For this review, take the finished solid that the model builds, in its own axes (mm). Face numbers are marked on the shaded views. A direction names the side the tool comes from. Coordinates: 2 decimals unless noted, no trailing zeros. Loops run counter-clockwise (first coordinate to the right, second up) from the corner with the lowest first, then second, coordinate; pieces in that order, holes last. Notation, with made-up numbers: M 1,-40 L 36,-40 A14 ccw 36,-31 Z; hole C -25,76.5 d2. An arc over 180 degrees is marked long. Answer as a JSON object with one key per item and string values. Group by question number.
Item 1: Tool access review of the marked faces 1 and 2: name each direction out of +Z, -Z, +X, -X, +Y, -Y from which nothing blocks a thin tool from reaching the whole face with its end or side.
Item 2: Insertion check: pin 1 (10 mm diameter, centred on x = -21, y = -33, fed in from +Z); pin 2 (4 mm diameter, centred on y = -14.5, z = 24.5, fed in from -X); pin 3 (1 mm diameter, centred on y = -13, z = 26, fed in from -X). Each pin has a flat end and moves straight along its axis. Give the tip position at first contact, or say it passes through.
Item 3: Wall thickness on L1, parallel to Y at x = -19.05, z = -1.75; L2, parallel to Z at x = -2.5, y = -26 (3 decimals); L3, parallel to X at y = -19, z = -1 (3 decimals): over which ranges is each line inside the solid? List them lowest first. Write a range as from..to.
Item 4: Add section B-B (z = 23.5). State the section outline as (x, y) points, then the cut area to 3 significant figures.
Item 5: Add section C-C (x = -27). State the section outline as (y, z) points (3 decimals).
Item 6: Add section A-A (x = -19.05). State the section outline as (y, z) points (3 decimals).
from build123d import *

# Parameters (mm, degrees)
SKETCH13_R              = 1.651
BASE_FLANGE5_DEPTH      = 3.175
EDGE_FLANGE4_START      = -51.763631849
EDGE_FLANGE4_DEPTH      = 40.665312179
CUT_EXTRUDE4_DEPTH      = 53.975
CUT_EXTRUDE4_DEPTH_BACK = 5.588


# Read off the part's stored shape, not the designer's step: Edge-Flange4
# Sheet-metal steps are written as plain solids
with BuildPart() as part:
    # Sketch13 → Base-Flange5 (new body)
    with BuildSketch(Plane.XY):
        Polygon((-31.75, 0), (0, 0), (0, -38.1), (-45.964697135, -38.1), align=None)
        with Locations((-19.05, -19.05)):
            Circle(SKETCH13_R, mode=Mode.SUBTRACT)
    extrude(amount=-BASE_FLANGE5_DEPTH)

    # Edge-Flange4 outline → Edge-Flange4 (add)
    with BuildSketch(Plane(origin=(0, 0, 0), x_dir=(0.9369164518419233, -0.34955337542060905, 0), z_dir=(0.34955337542060905, 0.9369164518419232, 0)).offset(EDGE_FLANGE4_START)):
        with BuildLine():
            Line((-29.747097346, -45.72), (-29.747097346, 3.175))
            ThreePointArc((-29.747097346, 3.175), (-31.992161376, 2.24506403), (-32.922097346, 0))
            Line((-32.922097346, 0), (-32.922097346, -45.72))
            Line((-32.922097346, -45.72), (-29.747097346, -45.72))
        make_face()
    extrude(amount=EDGE_FLANGE4_DEPTH)

    # Sketch51 → Cut-Extrude4 (cut, two sides: drawn at the far end of the back side and taken through both)
    with BuildSketch(Plane.XY.offset(-CUT_EXTRUDE4_DEPTH_BACK)):
        Polygon((-31.75, 0), (-35.138776015, 0), (-34.724709735, 1.109831967), align=None)
    extrude(amount=CUT_EXTRUDE4_DEPTH + CUT_EXTRUDE4_DEPTH_BACK, mode=Mode.SUBTRACT)


solid = part.part
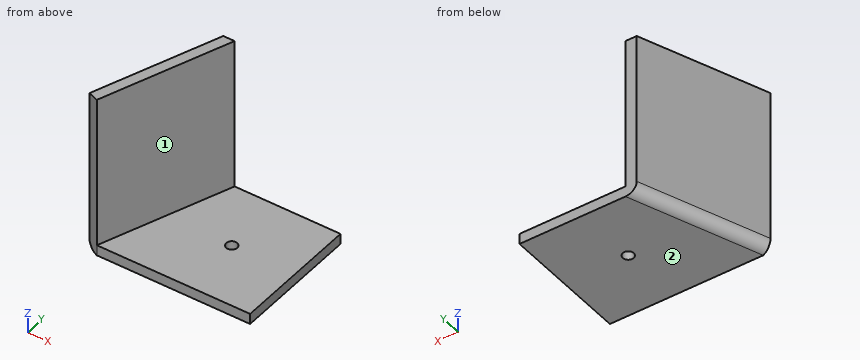
From the geometry:
{
 "1": {"face 1": "+Z, +X, -Y", "face 2": "-Z, +X, -X, +Y, -Y"},
 "2": {"pin 1": "stops at z = 0", "pin 2": "stops at x = -41.29", "pin 3": "stops at x = -40.18"},
 "3": {"L1": "y = -38.1..-20.7, -17.4..0", "L2": "z = -3.175..0", "L3": "x = -42.055..-20.7, -17.4..0"},
 "4": {"outline": "M -48.94,-36.99 L -45.96,-38.1 L -31.75,0 L -35.14,0 Z", "area": "127 mm²"},
 "5": {"outline": "M -38.1,-3.175 L 0,-3.175 L 0,0 L -38.1,0 Z"},
 "6": {"outline": "M -38.1,-3.175 L -20.701,-3.175 L -20.701,0 L -38.1,0 Z; M -17.399,-3.175 L 0,-3.175 L 0,0 L -17.399,0 Z"}
}
